Geometry check sheet. Reference: the model listing, model coordinates, mm. Face numbers are marked on the shaded views. Round coordinates to 2 decimals unless told otherwise and drop trailing zeros. Loops run counter-clockwise (first coordinate to the right, second up) from the corner with the lowest first, then second, coordinate; pieces in that order, holes last. Notation, with made-up numbers: (2, -8) - (14, -8) arc R14 ccw to (14, 13) - close; hole circle Ø1 at (69, -26.5). An arc over 180 degrees is marked (long way). Answer in a Markdown table with one row per item. Add a question column.
```python
from build123d import *

# Parameters (mm, degrees)
SKETCH1_W           = 50
SKETCH1_H           = 40
BOSS_EXTRUDE1_DEPTH = 5
SKETCH2_R           = 8
CUT_EXTRUDE1_DEPTH  = 5
CUT_EXTRUDE2_DEPTH  = 10
FILLET1_R           = 5
FILLET2_R           = 5


with BuildPart() as part:
    # Sketch1 → Boss-Extrude1 (new body)
    with BuildSketch(Plane.XY):
        with Locations((6.010513563, 6.766366312)):
            Rectangle(SKETCH1_W, SKETCH1_H)
    extrude(amount=BOSS_EXTRUDE1_DEPTH)

    # Sketch2 → Cut-Extrude1 (cut)
    with BuildSketch(Plane(origin=(0, 0, 0), x_dir=(-1, 0, 0), z_dir=(0, 0, -1))):
        with Locations((-18.760103176, 13.766366312)):
            Circle(SKETCH2_R)
        with Locations((6.739896824, 13.766366312)):
            Circle(SKETCH2_R)
    extrude(amount=-CUT_EXTRUDE1_DEPTH, mode=Mode.SUBTRACT)

    # Sketch3 → Cut-Extrude2 (cut)
    with BuildSketch(Plane.XY.offset(5)):
        Polygon((17.260103176, -13.233633688), (20.260103176, -13.233633688), (20.260103176, -7.233633688), (23.600103176, -7.233633688), (23.600103176, -4.233633688), (20.260103176, -4.233633688), (20.260103176, 0.766366312), (17.260103176, 0.766366312), (17.260103176, -4.233633688), (13.920103176, -4.233633688), (13.920103176, -7.233633688), (17.260103176, -7.233633688), align=None)
        Polygon((-8.239896824, -13.233633688), (-5.239896824, -13.233633688), (-5.239896824, -7.233633688), (-1.899896824, -7.233633688), (-1.899896824, -4.233633688), (-5.239896824, -4.233633688), (-5.239896824, 0.766366312), (-8.239896824, 0.766366312), (-8.239896824, -4.233633688), (-11.579896824, -4.233633688), (-11.579896824, -7.233633688), (-8.239896824, -7.233633688), align=None)
    extrude(amount=-CUT_EXTRUDE2_DEPTH, mode=Mode.SUBTRACT)

    # Fillet1
    fillet1_edges = [part.edges().sort_by_distance(p)[0] for p in [
        (-18.989486437, 26.766366312, 2.5),
    ]]
    fillet(fillet1_edges, radius=FILLET1_R)

    # Fillet2
    fillet2_edges = [part.edges().sort_by_distance(p)[0] for p in [
        (31.010513563, 26.766366312, 2.5),
    ]]
    fillet(fillet2_edges, radius=FILLET2_R)


solid = part.part
```
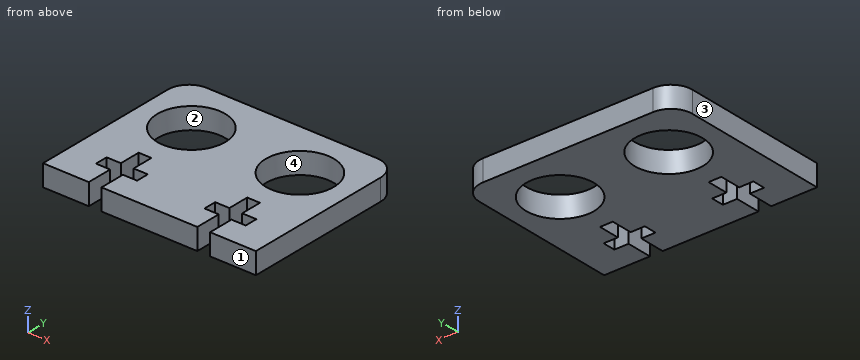
Q1. Cross-section at D-D, the plane z = 2.1. State how many separate pieces and enclosed holes the cut face has, plus the area to 3 significant figures.
Q2. Cross-section at B-B, the plane x = 16. Enter the section's corners in (y, z).
Q3. Depth check by flat-ended pin: P1, Ø0.9, axis at x = 18.5, z = 2, coming from the -Y side; P2, Ø4, axis at x = 19.5, y = 18, coming from the -Z side. Enter the tip coordinate at first touch or a pass-through.
Q4. Release check for a two-part mould opening along X. For the marked faces 1, 2, 3 and 4 record: +X half, -X half, draft (parallel to the pull), parting line (faces both ways), or undercut.
Q5. Scan lines: line 1 (X direction, y = -7.5, z = 3.2); line 2 (X direction, y = -5, z = 2.65); line 3 (Y direction, x = -11, z = 0.85) (3 decimals). Record each from-to range of solid material in increasing order. Write a range as from..to.
Q6. Cross-section at C-C, the plane x = -13. Enter the section's corners in (y, z), plus the area to 3 significant figures.
Q7. Cross-section at A-A, the plane y = -5. Enter the section's corners in (x, z), plus the area to 3 significant figures.
Check sheet entries:
| question | item | result |
|---|---|---|
| 1 | separate pieces | 1 |
| 1 | enclosed holes | 2 |
| 1 | area | 1,460 mm² |
| 2 | outline | (-13.23, 0) - (-7.23, 0) - (-7.23, 5) - (-13.23, 5) - close; (-4.23, 0) - (6.26, 0) - (6.26, 5) - (-4.23, 5) - close; (21.28, 0) - (26.77, 0) - (26.77, 5) - (21.28, 5) - close |
| 3 | P1 | y = 0.77 |
| 3 | P2 | through |
| 4 | face 1 | draft |
| 4 | face 2 | undercut |
| 4 | face 3 | -X half |
| 4 | face 4 | undercut |
| 5 | line 1 | -18.99..-8.24, -5.24..17.26, 20.26..31.01 |
| 5 | line 2 | -18.99..-11.58, -1.9..13.92, 23.6..31.01 |
| 5 | line 3 | -13.234..-7.234, -4.234..6.995, 20.538..26.766 |
| 6 | outline | (-13.23, 0) - (8.79, 0) - (8.79, 5) - (-13.23, 5) - close; (18.75, 0) - (26.77, 0) - (26.77, 5) - (18.75, 5) - close |
| 6 | area | 150 mm² |
| 7 | outline | (-18.99, 0) - (-11.58, 0) - (-11.58, 5) - (-18.99, 5) - close; (-1.9, 0) - (13.92, 0) - (13.92, 5) - (-1.9, 5) - close; (23.6, 0) - (31.01, 0) - (31.01, 5) - (23.6, 5) - close |
| 7 | area | 153 mm² |
